Check sheet for the drawn part. Datum: minimum x, y, z corner. Units: mm. Coordinates: 2 decimals unless noted, no trailing zeros. Order: outer loops, then holes, each group sorted by start corner. A loop starts at its lowest first (then second) coordinate and runs counter-clockwise, first axis right, second up. Notation, with made-up numbers: (-4, 7.5) -> (32, 7.5) arc R24 cw to (32, 33.5) -> close; hole circle Ø4 at (46.5, 54.5). An arc over 180 degrees is marked (long way). Answer as CSV lines item,"result".
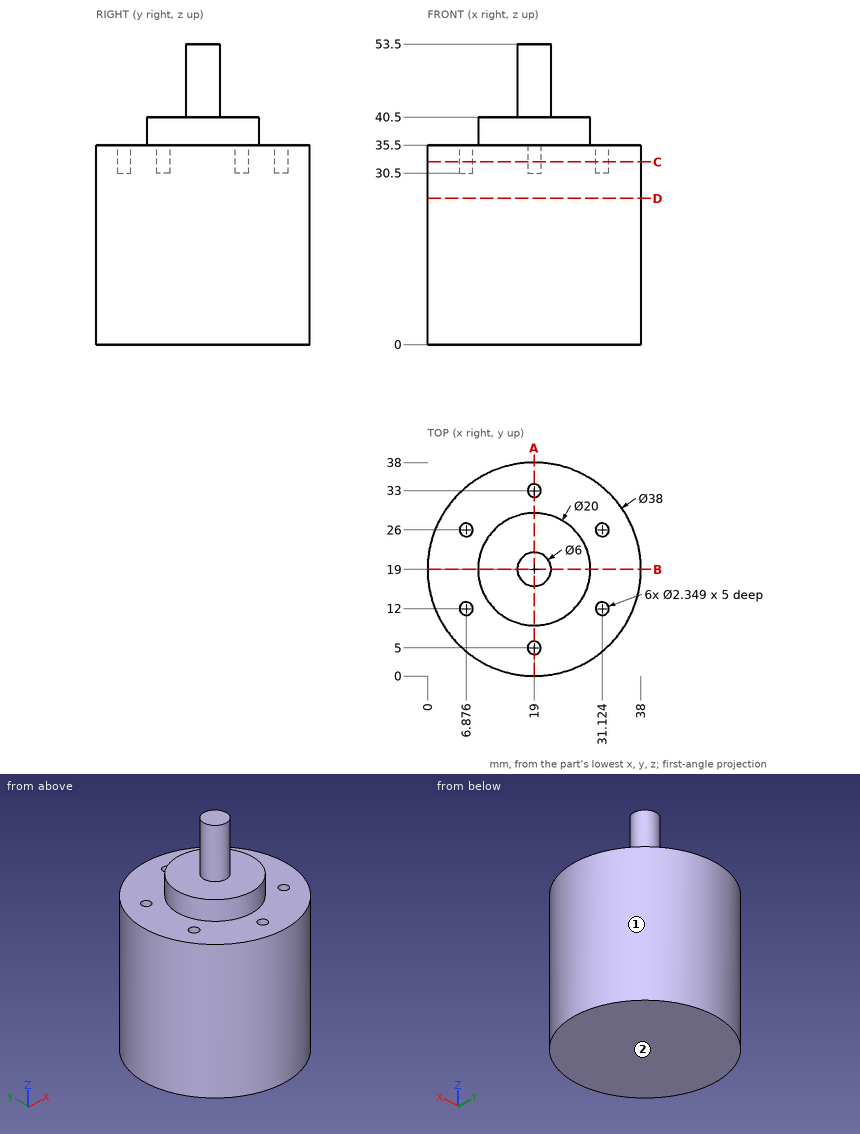
Item 1: Thickness scan on line 1 (Y direction, x = 19, z = 31.8) (1 decimal); line 2 (Y direction, x = 31, z = 35); line 3 (Z direction, x = 6, y = 10.5). Record the ranges inside material, lowest first.
Answer list:
line 1,"0 to 3.8, 6.2 to 31.8, 34.2 to 38"
line 2,"4.27 to 10.83, 13.17 to 24.83, 27.17 to 33.73"
line 3,"0 to 35.5"
Item 2: Depth check by flat-ended pin: pin 1 Ø1.9 at (x, y) = (6.5, 12) entering from +Z; pin 2 Ø2 at (x, y) = (6.88, 26) entering from +Z; pin 3 Ø1.5 at (y, z) = (13, 40) entering from +X. Enter the tip coordinate at first touch or a pass-through.
Answer list:
pin 1,"z = 35.5"
pin 2,"z = 30.5"
pin 3,"x = 27.51"
Item 3: Release check for a two-part mould opening along Y. For the marked faces 1 and 2 record: +Y half, -Y half, draft (parallel to the pull), parting line (faces both ways), or undercut.
Answer list:
face 1,"parting line"
face 2,"draft"
Item 4: Section check C-C, the plane z = 32.5. Record the boundary of the cut face in (x, y) (1 decimal).
Answer list:
outline,"circle Ø38 at (19, 19); hole circle Ø2.3 at (6.9, 12); hole circle Ø2.3 at (6.9, 26); hole circle Ø2.3 at (19, 5); hole circle Ø2.3 at (19, 33); hole circle Ø2.3 at (31.1, 12); hole circle Ø2.3 at (31.1, 26)"
Item 5: Section check A-A, the plane x = 19. Record the boundary of the cut face in (y, z) (1 decimal), plus the area to 3 significant figures.
Answer list:
outline,"(0, 0) -> (38, 0) -> (38, 35.5) -> (34.2, 35.5) -> (34.2, 30.5) -> (31.8, 30.5) -> (31.8, 35.5) -> (29, 35.5) -> (29, 40.5) -> (22, 40.5) -> (22, 53.5) -> (16, 53.5) -> (16, 40.5) -> (9, 40.5) -> (9, 35.5) -> (6.2, 35.5) -> (6.2, 30.5) -> (3.8, 30.5) -> (3.8, 35.5) -> (0, 35.5) -> close"
area,"1,500 mm2"
Item 6: Section check B-B, the plane y = 19. Record the boundary of the cut face in (x, z), plus the area to 3 significant figures.
Answer list:
outline,"(0, 0) -> (38, 0) -> (38, 35.5) -> (29, 35.5) -> (29, 40.5) -> (22, 40.5) -> (22, 53.5) -> (16, 53.5) -> (16, 40.5) -> (9, 40.5) -> (9, 35.5) -> (0, 35.5) -> close"
area,"1,530 mm2"
Item 7: Section check D-D, the plane z = 26. Record the boundary of the cut face in (x, y).
Answer list:
outline,"circle Ø38 at (19, 19)"
